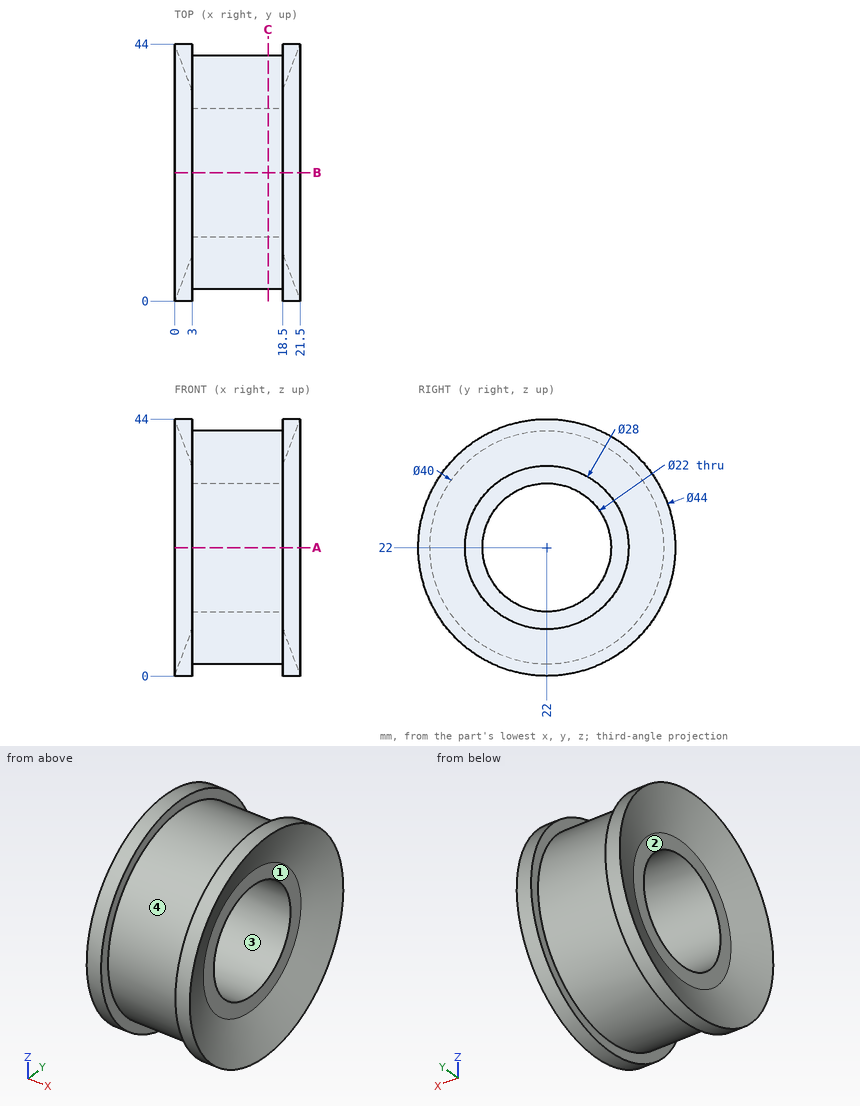
Geometry check sheet. Reference: drawing and pictorial views, mm from the part's lowest x, y, z. A direction names the side the tool comes from. Coordinates: 2 decimals unless noted, no trailing zeros. Order: outer loops, then holes, each group sorted by start corner. A loop starts at its lowest first (then second) coordinate and runs counter-clockwise, first axis right, second up. Notation, with made-up numbers: M 55.5,-25 L 110.5,-25 A8 cw 110.5,-17 Z; hole C 27.5,60 d8. An arc over 180 degrees is marked long. Return JSON: item names as keys, results as strings.
1) Cross-section at C-C, the plane x = 16. Record the boundary of the cut face in (y, z), and give its area (3 significant figures).
Answer list:
{"outline": "C 22,22 d40; hole C 22,22 d22", "area": "877 mm2"}
2) Cross-section at A-A, the plane z = 22. Record the boundary of the cut face in (x, y).
Answer list:
{"outline": "M 0,0 L 3,0 L 3,2 L 18.5,2 L 18.5,0 L 21.5,0 L 18.5,8 L 18.5,11 L 3,11 L 3,8 Z; M 0,44 L 3,36 L 3,33 L 18.5,33 L 18.5,36 L 21.5,44 L 18.5,44 L 18.5,42 L 3,42 L 3,44 Z"}
3) Gauge pin test, flat ends, axial feed: pin 1 (12 mm diameter, centred on x = 10.5, z = 9, fed in from -Y) (3 decimals); pin 2 (3 mm diameter, centred on y = 19.5, z = 12, fed in from +X); pin 3 (8 mm diameter, centred on x = 10.5, y = 30, fed in from -Z). Record the tip position at first contact, or that the pin passes through.
Answer list:
{"pin 1": "y = 3.265", "pin 2": "x = 18.5", "pin 3": "z = 2.4"}
4) Release check for a two-part mould opening along Z. For the marked faces 3 and 4 record: +Z half, -Z half, draft (parallel to the pull), parting line (faces both ways), or undercut.
Answer list:
{"face 3": "undercut", "face 4": "parting line"}
5) Thickness scan on L1, parallel to Y at x = 8, z = 22; L2, parallel to X at y = 28.5, z = 11.5; L3, parallel to Z at x = 9.75, y = 14.5. Record the ranges inside material, lowest first. Write a range as [from, to].
Answer list:
{"L1": "[2, 11], [33, 42]", "L2": "[3, 18.5]", "L3": "[3.46, 13.95], [30.05, 40.54]"}
6) Access from +Z, -Z, +X, -X, +Y, -Y to the whole of each face (thin tool, end or side, straight path). Record for the marked faces 1 and 2.
Answer list:
{"face 1": "+X", "face 2": "-X"}
